The listing builds one solid part. Answer for the finished solid, in the listing's coordinates (mm). A direction names the side the tool comes from. Coordinates: 2 decimals unless noted, no trailing zeros. Loops run counter-clockwise (first coordinate to the right, second up) from the corner with the lowest first, then second, coordinate; pieces in that order, holes last. Notation, with made-up numbers: (-2.75, 11) -> (53.25, 11) arc R15 ccw to (53.25, 34) -> close; hole circle Ø10 at (74, 1.25). An arc over 180 degrees is marked (long way). Answer in a Markdown table with one row per item.
```python
from build123d import *

# Parameters (mm, degrees)
F0_R     = 1.5
F1_DEPTH = 3
F3_DEPTH = 16
F4_R     = 5
F5_W     = 5
F5_H     = 5
F6_DEPTH = 1


with BuildPart() as f1:
    # F0 (on Top) → F1 (new body)
    with BuildSketch(Plane.XY):
        Polygon((30, -35), (30, 35), (22, 35), (22, 22), (-11, 22), (-11, 35), (-30, 35), (-30, -35), align=None)
        with Locations((-24.5, -29)):
            Circle(F0_R, mode=Mode.SUBTRACT)
        with Locations((24.5, -29)):
            Circle(F0_R, mode=Mode.SUBTRACT)
        with Locations((-24.5, 29)):
            Circle(F0_R, mode=Mode.SUBTRACT)
        with Locations((24.5, 29)):
            Circle(F0_R, mode=Mode.SUBTRACT)
    extrude(amount=-F1_DEPTH)

    # F2 (on face) → F3 (join)
    with BuildSketch(Plane(origin=(0, 0, -3), x_dir=(1, 0, 0), z_dir=(0, 0, -1))):
        Polygon((27, -26.5), (22, -26.5), (22, -31.5), (23, -31.5), (23, -29), (23, -27.5), (24.5, -27.5), (27, -27.5), align=None)
        Polygon((-22, -31.5), (-22, -26.5), (-27, -26.5), (-27, -27.5), (-24.5, -27.5), (-23, -27.5), (-23, -29), (-23, -31.5), align=None)
        Polygon((-27, 26.5), (-22, 26.5), (-22, 31.5), (-23, 31.5), (-23, 29), (-23, 27.5), (-24.5, 27.5), (-27, 27.5), align=None)
        Polygon((22, 31.5), (22, 26.5), (27, 26.5), (27, 27.5), (24.5, 27.5), (23, 27.5), (23, 29), (23, 31.5), align=None)
    extrude(amount=F3_DEPTH)

    # F4
    f4_edges = [f1.edges().sort_by_distance(p)[0] for p in [
        (-30, 35, -1.5),
        (-30, -35, -1.5),
        (-11, 35, -1.5),
        (-11, 22, -1.5),
        (22, 22, -1.5),
        (30, -35, -1.5),
    ]]
    fillet(f4_edges, radius=F4_R)

    # F5 (on face) → F6 (join)
    with BuildSketch(Plane(origin=(0, 0, -19), x_dir=(1, 0, 0), z_dir=(0, 0, -1))):
        with Locations((-24.5, 29)):
            Rectangle(F5_W, F5_H)
        with BuildLine():
            ThreePointArc((-24.5, 27.5), (-25.56066, 30.06066), (-23, 29))
            ThreePointArc((-23, 29), (-23.43934, 27.93934), (-24.5, 27.5))
        make_face(mode=Mode.SUBTRACT)
        with Locations((24.5, 29)):
            Rectangle(F5_W, F5_H)
        with BuildLine():
            ThreePointArc((24.5, 27.5), (23.43934, 27.93934), (23, 29))
            ThreePointArc((23, 29), (25.56066, 30.06066), (24.5, 27.5))
        make_face(mode=Mode.SUBTRACT)
        with Locations((24.474937, -29)):
            Rectangle(F5_W, F5_H)
        with BuildLine():
            ThreePointArc((24.5, -27.5), (25.56066, -30.06066), (23, -29))
            ThreePointArc((23, -29), (23.43934, -27.93934), (24.5, -27.5))
        make_face(mode=Mode.SUBTRACT)
        with Locations((-24.5, -29)):
            Rectangle(F5_W, F5_H)
        with BuildLine():
            ThreePointArc((-24.5, -27.5), (-23.43934, -27.93934), (-23, -29))
            ThreePointArc((-23, -29), (-25.56066, -30.06066), (-24.5, -27.5))
        make_face(mode=Mode.SUBTRACT)
    extrude(amount=F6_DEPTH)


solid = f1.part
```
Item 1: A cutting plane is placed at B-B, the plane z = -1.25. Determine the outline of the cut face in (x, y).
Findings below:
| item | result |
|---|---|
| outline | (-30, -30) arc R5 ccw to (-25, -35) -> (25, -35) arc R5 ccw to (30, -30) -> (30, 35) -> (22, 35) -> (22, 27) arc R5 cw to (17, 22) -> (-6, 22) arc R5 cw to (-11, 27) -> (-11, 30) arc R5 ccw to (-16, 35) -> (-25, 35) arc R5 ccw to (-30, 30) -> close; hole circle Ø3 at (-24.5, -29); hole circle Ø3 at (-24.5, 29); hole circle Ø3 at (24.5, -29); hole circle Ø3 at (24.5, 29) |
Item 2: A cutting plane is placed at D-D, the plane y = -13. Determine the outline of the cut face in (x, z), plus the area to 3 significant figures.
Findings below:
| item | result |
|---|---|
| outline | (-30, -3) -> (30, -3) -> (30, 0) -> (-30, 0) -> close |
| area | 180 mm2 |
Item 3: Find the intervals of material crossed by probe 1 along X at (y, z) = (29, -2.4); probe 2 along Y at (x, z) = (24.5, -1.15); probe 3 along X at (y, z) = (-29, -19.65), in increasing order.
Findings below:
| item | result |
|---|---|
| probe 1 | x = -30 to -26, -23 to -11, 22 to 23, 26 to 30 |
| probe 2 | y = -35 to -30.5, -27.5 to 27.5, 30.5 to 35 |
| probe 3 | x = -27 to -26, -23 to -22, 22 to 23, 26 to 27 |
Item 4: A cutting plane is placed at C-C, the plane x = 5.5. Determine the outline of the cut face in (y, z).
Findings below:
| item | result |
|---|---|
| outline | (-35, -3) -> (22, -3) -> (22, 0) -> (-35, 0) -> close |
Item 5: A tool of negligible diameter and unlimited length cuts with its end or side. For faces 4 (the face through (-23, 29, -11)), 5 (the face through (-22.8, -31.5, -13.3)), from which of +Z, -Z, +X, -X, +Y, -Y can it reach the whole face along a straight path? Write none if from no direction.
Findings below:
| item | result |
|---|---|
| face 4 | -X, +Y |
| face 5 | -Z, +X, -X, -Y |
Item 6: Determine the mould class of faces 1 (the face through (24, -26.5, -11)), 2 (the face through (-23.3, -27.8, -19)), 3 (the face through (-20, 35, -1)) for opening direction Y: +Y half, -Y half, draft (parallel to the pull), parting line (faces both ways), or undercut.
Findings below:
| item | result |
|---|---|
| face 1 | undercut |
| face 2 | draft |
| face 3 | +Y half |
Item 7: Flat-ended cylindrical pins translate along their axes: pin 1 Ø5 at (x, y) = (-24.5, 29) entering from +Z; pin 2 Ø1.5 at (x, y) = (-4.5, 13) entering from -Z; pin 3 Ø5.5 at (x, z) = (23.5, -10) entering from +Y; pin 4 Ø1.2 at (y, z) = (28.5, -9) entering from +X. Find the tip coordinate at first contact, or state that the pin passes through.
Findings below:
| item | result |
|---|---|
| pin 1 | stops at z = 0 |
| pin 2 | stops at z = -3 |
| pin 3 | stops at y = 31.5 |
| pin 4 | stops at x = 23 |
Item 8: A cutting plane is placed at A-A, the plane z = -11.75. Determine the outline of the cut face in (x, y), plus the area to 3 significant figures.
Findings below:
| item | result |
|---|---|
| outline | (-27, -27.5) -> (-23, -27.5) -> (-23, -31.5) -> (-22, -31.5) -> (-22, -26.5) -> (-27, -26.5) -> close; (-27, 26.5) -> (-22, 26.5) -> (-22, 31.5) -> (-23, 31.5) -> (-23, 27.5) -> (-27, 27.5) -> close; (21.97, 26.5) -> (27, 26.5) -> (27, 27.5) -> (23, 27.5) -> (23, 31.5) -> (22, 31.5) -> (22, 27) arc R5 cw to start; (22, -31.5) -> (23, -31.5) -> (23, -27.5) -> (27, -27.5) -> (27, -26.5) -> (22, -26.5) -> close |
| area | 36.0 mm2 |
